```python
from build123d import *

# Parameters (mm, degrees)
SKETCH_1_W          = 24
SKETCH_1_H          = 24
EXTRUDE_1_DEPTH     = 12
FILLET_1_R          = 6
SKETCH_3_R          = 1.6
CUT_EXTRUDE_1_DEPTH = 9
SKETCH_4_R          = 3
CUT_EXTRUDE_2_DEPTH = 3
SKETCH_5_R          = 1.55
CUT_EXTRUDE_3_DEPTH = 23
SKETCH_7_R          = 16
EXTRUDE_2_DEPTH     = 2
EXTRUDE_START       = 2
SKETCH_8_R          = 16
EXTRUDE_3_DEPTH     = 2
SKETCH_9_R          = 2.55
CUT_EXTRUDE_4_DEPTH = 22
FILLET_2_R          = 0.2
FILLET_3_R          = 0.4


with BuildPart() as part:
    # 草图1 → 凸台-拉伸1 (new body)
    with BuildSketch(Plane(origin=(0, 0, 0), x_dir=(0, 0, -1), z_dir=(1, 0, 0))):
        with Locations((-12, 12)):
            Rectangle(SKETCH_1_W, SKETCH_1_H)
    extrude(amount=EXTRUDE_1_DEPTH)

    # 圆角1
    fillet_1_edges = [part.edges().sort_by_distance(p)[0] for p in [
        (6, 0, 0),
        (6, 0, 24),
        (6, 24, 24),
        (6, 24, 0),
    ]]
    fillet(fillet_1_edges, radius=FILLET_1_R)

    # 草图3 → 切除-拉伸1 (cut)
    with BuildSketch(Plane(origin=(0, 24, 0), x_dir=(1, 0, 0), z_dir=(0, 1, 0))):
        with Locations(Location((6, -12, 0), (0, 0, 270))):
            Circle(SKETCH_3_R)
    extrude(amount=-CUT_EXTRUDE_1_DEPTH, mode=Mode.SUBTRACT)

    # 草图4 → 切除-拉伸2 (cut)
    with BuildSketch(Plane(origin=(0, 24, 0), x_dir=(1, 0, 0), z_dir=(0, 1, 0))):
        with Locations(Location((6, -12, 0), (0, 0, 270))):
            Circle(SKETCH_4_R)
    extrude(amount=-CUT_EXTRUDE_2_DEPTH, mode=Mode.SUBTRACT)

    # 草图5 → 切除-拉伸3 (cut)
    with BuildSketch(Plane.ZY):
        with Locations((12, 12)):
            Circle(SKETCH_5_R)
    extrude(amount=-CUT_EXTRUDE_3_DEPTH, mode=Mode.SUBTRACT)

    # 草图7 → 凸台-拉伸2 (add)
    with BuildSketch(Plane(origin=(12, 0, 0), x_dir=(0, 0, -1), z_dir=(1, 0, 0))):
        with Locations((-12, 12)):
            Circle(SKETCH_7_R)
    extrude(amount=EXTRUDE_2_DEPTH)

    # 草图8 → 凸台-拉伸3 (add)
    with BuildSketch(Plane.ZY.offset(EXTRUDE_START)):
        with Locations(Location((12, 12, 0), (0, 0, 180))):
            Circle(SKETCH_8_R)
    extrude(amount=-EXTRUDE_3_DEPTH)

    # 草图9 → 切除-拉伸4 (cut)
    with BuildSketch(Plane.ZY.offset(2)):
        with Locations((12, 12)):
            Circle(SKETCH_9_R)
    extrude(amount=-CUT_EXTRUDE_4_DEPTH, mode=Mode.SUBTRACT)

    # 圆角2
    fillet_2_edges = [part.edges().sort_by_distance(p)[0] for p in [
        (6, 21, 10.4),
    ]]
    fillet(fillet_2_edges, radius=FILLET_2_R)

    # 圆角3
    fillet_3_edges = [part.edges().sort_by_distance(p)[0] for p in [
        (14, 12, 9.45),
        (-2, 12, 9.45),
    ]]
    fillet(fillet_3_edges, radius=FILLET_3_R)


solid = part.part
```
Geometry check sheet. Reference: the model listing, model coordinates, mm. A direction names the side the tool comes from. Give positions to 0.01 mm unless a question says otherwise; leave off trailing zeros. Order: outer loops, then holes, each group sorted by start corner. A loop starts at its lowest first (then second) coordinate and runs counter-clockwise, first axis right, second up.
1. Thickness scan on L1, parallel to X at y = 26, z = 19; L2, parallel to X at y = 18, z = 12; L3, parallel to Z at x = 3, y = 6. Record the ranges inside material, lowest first.
2. Section check B-B, the plane y = 12. Enter the section's corners in (x, z).
3. Gauge pin test, flat ends, axial feed: pin 1 Ø1 at (x, z) = (5.5, 11.5) entering from +Y; pin 2 Ø1.5 at (x, z) = (11.5, 18) entering from -Y; pin 3 Ø3.5 at (x, z) = (6, 12) entering from +Y; pin 4 Ø6 at (y, z) = (12, 12) entering from -X. Record the tip position at first contact, or that the pin passes through.
4. Access from +Z, -Z, +X, -X, +Y, -Y to the whole of each face (thin tool, end or side, straight path). Record for faces 4 (the face through (6.084, 1.711, 1.804)), 5 (the face through (4.2, 22.5, 9.6)), 6 (the face through (6, 12, 24)), 7 (the face through (3, 24, 13)).
5. Section check D-D, the plane y = 17. Enter the section's corners in (x, z).
6. Section check C-C, the plane x = 6. Enter the section's corners in (y, z), and give its area (3 significant figures).
7. Release check for a two-part mould opening along Z. For faces 1 (the face through (-1.014, 21.736, 24.697)), 2 (the face through (6, 15, 12)), 3 (the face through (6.084, 22.196, 1.711)) record: pulls with the +Z half, pulls with the -Z half, needs draft (parallel to the pull), parting line crosses it, or undercut.
Values follow:
1. L1: x = -2 to 0, 12 to 14
1. L2: x = -2 to 4.4, 7.6 to 14
1. L3: z = 0 to 24
2. outline: (-2, -4) - (0, -4) - (0, 0) - (12, 0) - (12, -4) - (14, -4) - (14, 9.05) arc R0.4 ccw to (13.6, 9.45) - (-1.6, 9.45) arc R0.4 ccw to (-2, 9.05) - close; (-2, 14.95) arc R0.4 ccw to (-1.6, 14.55) - (13.6, 14.55) arc R0.4 ccw to (14, 14.95) - (14, 28) - (12, 28) - (12, 24) - (0, 24) - (0, 28) - (-2, 28) - close
3. pin 1: stops at y = 15
3. pin 2: stops at y = -3.05
3. pin 3: stops at y = 20.99
3. pin 4: stops at x = -2
4. face 4: -Z, -Y
4. face 5: +Y
4. face 6: +Z, +Y, -Y
4. face 7: +Z, -Z, +Y
5. outline: (-2, -3.2) - (0, -3.2) - (0, 0) - (12, 0) - (12, -3.2) - (14, -3.2) - (14, 27.2) - (12, 27.2) - (12, 24) - (0, 24) - (0, 27.2) - (-2, 27.2) - close; hole circle Ø3.2 at (6, 12)
6. outline: (0, 6) arc R6 ccw to (6, 0) - (18, 0) arc R6 ccw to (24, 6) - (24, 9) - (21, 9) - (21, 10.2) arc R0.2 ccw to (20.8, 10.4) - (15, 10.4) - (15, 13.6) - (20.8, 13.6) arc R0.2 ccw to (21, 13.8) - (21, 15) - (24, 15) - (24, 18) arc R6 ccw to (18, 24) - (6, 24) arc R6 ccw to (0, 18) - close; hole circle Ø5.1 at (12, 12)
6. area: 487 mm2
7. face 1: parting line crosses it
7. face 2: undercut
7. face 3: pulls with the -Z half
